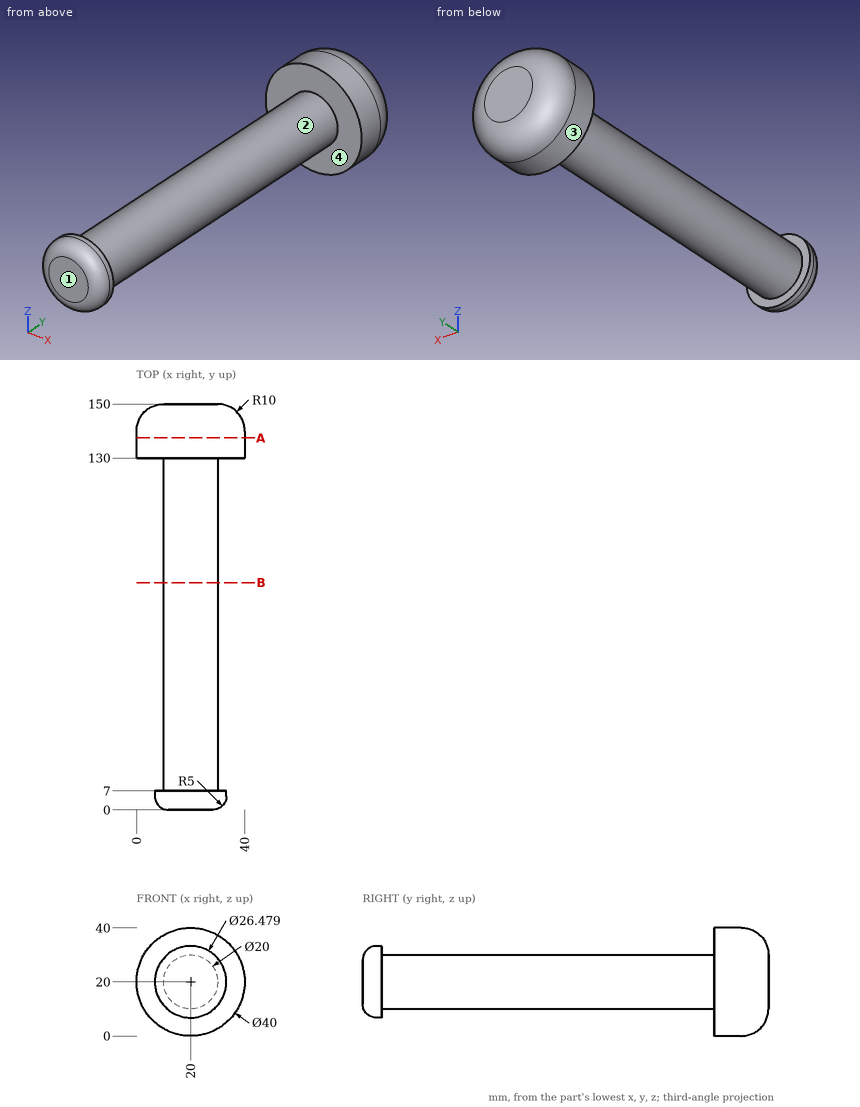
Can you work these out from the drawing? Everything is in mm from the part's minimum corner. Give positions to 0.01 mm unless a question says otherwise; leave off trailing zeros. Loops run counter-clockwise (first coordinate to the right, second up) from the corner with the lowest first, then second, coordinate; pieces in that order, holes last. Notation, with made-up numbers: (-22.75, -33) -> (-1.75, -33) arc R26 cw to (-1.75, -11) -> close; hole circle Ø2 at (76.5, 47.25). An arc over 180 degrees is marked (long way). Write item = value, one per line.
1) Suppose I cut it at B-B on y = 84. Write out the boundary of the cut face in (x, z), then the cut area to 3 significant figures.
Check result:
outline = circle Ø20 at (20, 20)
area = 314 mm2
2) Thinking about a two-plate mould opening in Y: for the marked faces 1, 2, 3 and 4, which applies, released by +Y, released by -Y, zero draft, split by the parting line, or undercut?
Check result:
face_1 = released by -Y
face_2 = undercut
face_3 = zero draft
face_4 = undercut
3) I need wall thicknesses on L1, parallel to Z at x = 20.5, y = 93.5; L2, parallel to Y at x = 31, z = 28; L3, parallel to X at y = 140.5, z = 28. Which ranges of each line are inside material? Lowest first, please. Write a range as from..to.
Check result:
L1 = 10.01..29.99
L2 = 130..149.33
L3 = 1.68..38.32
4) Suppose I cut it at A-A on y = 137.5. Write out the boundary of the cut face in (x, z).
Check result:
outline = circle Ø40 at (20, 20)
5) Will these pins go through, and if not, where does the flat tip stop? pin 1 (1 mm diameter, centred on x = 12, y = 131.5, fed in from -Z); pin 2 (2 mm diameter, centred on x = 29.5, y = 42.5, fed in from -Z); pin 3 (4 mm diameter, centred on x = 9.5, z = 17, fed in from -Y).
Check result:
pin_1 = 1.46
pin_2 = 14.73
pin_3 = 0.05
